Verification items for the finished model (mm, model axes). Face numbers are marked on the shaded views. A direction names the side the tool comes from. Coordinates: 2 decimals unless noted, no trailing zeros. Write each loop counter-clockwise with the first axis right and the second up, starting at its lowest first coordinate (ties: lowest second). Pieces come first, ordered by that corner, then holes. Notation, with made-up numbers: (27, 20.5) -> (55, 20.5) arc R18 ccw to (55, 54.5) -> close; hole circle Ø5 at (58, 84.5). An arc over 180 degrees is marked (long way). Answer in a Markdown table with one row per item.
```python
from build123d import *

# Parameters (mm, degrees)
F0_W      = 53
F0_H      = 63
F1_DEPTH  = 25
F2_W      = 51
F2_H      = 61
F3_DEPTH  = 24
F4_W      = 5
F4_H      = 5
F5_DEPTH  = 24
F6_R      = 1.5
F7_DEPTH  = 15
F8_R      = 2
F8_R_2    = 1
F9_DEPTH  = 5
F10_DEPTH = 1
F11_R     = 2
F12_R     = 2
F13_R     = 2
F14_R     = 2
F15_W     = 18.4732184559
F15_H     = 4
F16_DEPTH = 1
F17_W     = 10
F17_H     = 15
F18_DEPTH = 1
F19_W     = 10
F19_H     = 8
F20_DEPTH = 1
F21_DEPTH = 15
F22_R     = 2
F22_R_2   = 1
F23_DEPTH = 5


with BuildPart() as f1:
    # F0 (on Top) → F1 (new body)
    with BuildSketch(Plane.XY):
        with Locations((-36.9371324778, 48.9509678861)):
            Rectangle(F0_W, F0_H)
    extrude(amount=F1_DEPTH)

    # F2 (on face) → F3 (cut)
    with BuildSketch(Plane.XY.offset(25)):
        with Locations((-36.9371324778, 48.9509678861)):
            Rectangle(F2_W, F2_H)
    extrude(amount=-F3_DEPTH, mode=Mode.SUBTRACT)

    # F4 (on face) → F5 (join)
    with BuildSketch(Plane.XY.offset(1)):
        with Locations((-36.9371324778, 76.9509678861)):
            Rectangle(F4_W, F4_H)
        with Locations((-59.9371324778, 20.9509678861)):
            Rectangle(F4_W, F4_H)
        with Locations((-13.9371324778, 20.9509678861)):
            Rectangle(F4_W, F4_H)
    extrude(amount=F5_DEPTH)

    # F6 (on face) → F7 (cut)
    with BuildSketch(Plane.XY.offset(25)):
        with Locations((-36.9371324778, 76.9509678861)):
            Circle(F6_R)
        with Locations((-59.9371324778, 20.9509678861)):
            Circle(F6_R)
        with Locations((-13.9371324778, 20.9509678861)):
            Circle(F6_R)
    extrude(amount=-F7_DEPTH, mode=Mode.SUBTRACT)

    # F8 (on face) → F9 (join)
    with BuildSketch(Plane.XY.offset(1)):
        with Locations((-51.4371324778, 63.4509678861)):
            Circle(F8_R)
        with Locations((-51.4371324778, 63.4509678861)):
            Circle(F8_R_2, mode=Mode.SUBTRACT)
        with Locations((-17.4371324778, 29.4509678861)):
            Circle(F8_R)
        with Locations((-17.4371324778, 29.4509678861)):
            Circle(F8_R_2, mode=Mode.SUBTRACT)
    extrude(amount=F9_DEPTH)

    # F10 (cut): faces of the model
    f10_faces = [f1.faces().sort_by_distance(p)[0] for p in [
        (-51.4371324778, 63.4509678861, 1),
        (-17.4371324778, 29.4509678861, 1),
    ]]
    extrude(f10_faces, amount=-F10_DEPTH, mode=Mode.SUBTRACT)

    # F11
    f11_edges = [f1.edges().sort_by_distance(p)[0] for p in [
        (-63.437132, 80.450968, 12.5),
        (-10.437132, 80.450968, 12.5),
        (-10.437132, 17.450968, 12.5),
        (-63.437132, 17.450968, 12.5),
        (-39.437132, 74.450968, 13),
        (-34.437132, 74.450968, 13),
        (-39.437132, 79.450968, 13),
        (-34.437132, 79.450968, 13),
        (-62.437132, 23.450968, 13),
        (-57.437132, 18.450968, 13),
        (-16.437132, 18.450968, 13),
        (-11.437132, 23.450968, 13),
    ]]
    fillet(f11_edges, radius=F11_R)

    # F12
    f12_edges = [f1.edges().sort_by_distance(p)[0] for p in [
        (-57.437132, 23.450968, 13),
        (-16.437132, 23.450968, 13),
    ]]
    fillet(f12_edges, radius=F12_R)

    # F13
    f13_edges = [f1.edges().sort_by_distance(p)[0] for p in [
        (-62.437132, 79.450968, 13),
    ]]
    fillet(f13_edges, radius=F13_R)

    # F14
    f14_edges = [f1.edges().sort_by_distance(p)[0] for p in [
        (-11.437132, 79.450968, 13),
    ]]
    fillet(f14_edges, radius=F14_R)

    # F15 (on face) → F16 (cut)
    with BuildSketch(Plane.XZ.offset(-79.4509678861)):
        with Locations((-51.2005232498, 11)):
            Rectangle(F15_W, F15_H)
    extrude(amount=-F16_DEPTH, mode=Mode.SUBTRACT)

    # F17 (on face) → F18 (cut)
    with BuildSketch(Plane.XZ.offset(-17.4509678861)):
        with Locations((-38.4371324778, 17.5)):
            Rectangle(F17_W, F17_H)
    extrude(amount=-F18_DEPTH, mode=Mode.SUBTRACT)

    # F19 (on face) → F20 (cut)
    with BuildSketch(Plane.YZ.offset(-10.4371324778)):
        with Locations((67.9509678861, 10)):
            Rectangle(F19_W, F19_H)
    extrude(amount=-F20_DEPTH, mode=Mode.SUBTRACT)

    # F21 (cut): faces of the model
    f21_faces = [f1.faces().sort_by_distance(p)[0] for p in [
        (-59.9371324778, 20.9509678861, 10),
        (-13.9371324778, 20.9509678861, 10),
        (-36.9371324778, 76.9509678861, 10),
    ]]
    extrude(f21_faces, amount=-F21_DEPTH, mode=Mode.SUBTRACT)

    # F22 (on face) → F23 (join)
    with BuildSketch(Plane.XY.offset(1)):
        with Locations((-28.4371324778, 66.9157579541)):
            Circle(F22_R)
        with Locations((-28.4371324778, 66.9157579541)):
            Circle(F22_R_2, mode=Mode.SUBTRACT)
    extrude(amount=F23_DEPTH)


solid = f1.part
```
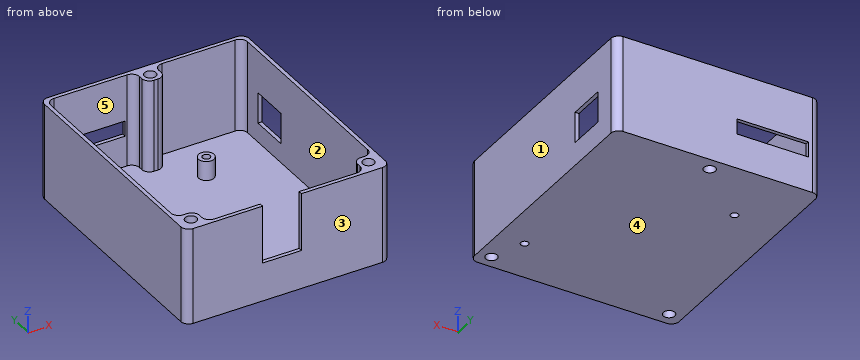
1. Sectioned sample at B-B, the plane y = 60. Record the cut outline in (x, z).
Findings below:
| item | result |
|---|---|
| outline | (-63.44, 0) -> (-10.44, 0) -> (-10.44, 25) -> (-11.44, 25) -> (-11.44, 1) -> (-62.44, 1) -> (-62.44, 25) -> (-63.44, 25) -> close |
2. Sectioned sample at C-C, the plane z = 20.25. Count the separate pieces of the cut face and the enclosed holes in it, and give its area (3 significant figures).
Findings below:
| item | result |
|---|---|
| separate pieces | 1 |
| enclosed holes | 3 |
| area | 272 mm² |
3. Release check for a two-part mould opening along Y. For the marked faces 1, 2 and 3 record: released by +Y, released by -Y, zero draft, split by the parting line, or undercut.
Findings below:
| item | result |
|---|---|
| face 1 | zero draft |
| face 2 | undercut |
| face 3 | released by -Y |
4. Access from +Z, -Z, +X, -X, +Y, -Y to the whole of each face (thin tool, end or side, straight path). Record for the marked faces 4 and 5.
Findings below:
| item | result |
|---|---|
| face 4 | -Z, +X, -X, +Y, -Y |
| face 5 | +Z |
5. Sectioned sample at A-A, the plane x = -54.5. Record the cut outline in (y, z), and give its area (3 significant figures).
Findings below:
| item | result |
|---|---|
| outline | (17.45, 0) -> (80.45, 0) -> (80.45, 9) -> (79.45, 9) -> (79.45, 1) -> (18.45, 1) -> (18.45, 25) -> (17.45, 25) -> close; (79.45, 13) -> (80.45, 13) -> (80.45, 25) -> (79.45, 25) -> close |
| area | 107 mm² |
6. Material ranges on probe 1 along Y at (x, z) = (-51.5, 23.75); probe 2 along X at (y, z) = (20.5, 3); probe 3 along X at (y, z) = (53, 2.75), recorded low to high. Write a range as from..to.
Findings below:
| item | result |
|---|---|
| probe 1 | y = 17.45..18.45, 79.45..80.45 |
| probe 2 | x = -63.44..-61.37, -58.51..-57.44, -16.44..-15.37, -12.51..-10.44 |
| probe 3 | x = -63.44..-62.44, -11.44..-10.44 |
7. Go/stop test with flat-tipped pins: pin 1 (1.2 mm diameter, centred on x = -17.5, y = 29.5, fed in from +Z); pin 2 (3.5 mm diameter, centred on x = -59.94, y = 20.95, fed in from -Z); pin 3 (3 mm diameter, centred on x = -23, y = 42.5, fed in from +Z); pin 4 (0.8 mm diameter, centred on x = -11, z = 11, fed in from -Y). Record where each tip stops, or that it passes through.
Findings below:
| item | result |
|---|---|
| pin 1 | passes through |
| pin 2 | stops at z = 0 |
| pin 3 | stops at z = 1 |
| pin 4 | stops at y = 17.74 |
